Source: CAD feature listing. Evaluate the final solid. Frame: model axes, mm. Face numbers are marked on the shaded views. A direction names the side the tool comes from. Round coordinates to 2 decimals unless told otherwise and drop trailing zeros. Put each result on its own line as item: value.
```python
from build123d import *

# Parameters (mm, degrees)
SKETCH2_W               = 508
SKETCH2_H               = 127
BOSS_EXTRUDE1_DEPTH     = 63.5
SKETCH3_W               = 127
SKETCH3_H               = 127
BOSS_EXTRUDE2_DEPTH     = 444.5
SKETCH4_W               = 31.75
SKETCH4_H               = 31.75
CUT_EXTRUDE1_DEPTH      = 38.1
SKETCH5_R               = 12.7
CUT_EXTRUDE2_DEPTH      = 50.8
BOSS_EXTRUDE3_DEPTH     = 6.35
EXTRUDE_THIN1_START     = -6.35
EXTRUDE_THIN1_DEPTH     = 6.35
BOSS_EXTRUDE4_DEPTH     = 127
FILLET1_R               = 63.5
CUT_EXTRUDE3_DEPTH      = 583.156936495
CUT_EXTRUDE3_DEPTH_BACK = 583.156936495
SKETCH13_R              = 12.7


# Read off the part's stored shape, not the designer's step: Extrude-Thin1
with BuildPart() as part:
    # Sketch2 → Boss-Extrude1 (new body)
    with BuildSketch(Plane(origin=(0, 0, 0), x_dir=(0, 0, -1), z_dir=(1, 0, 0))):
        Rectangle(SKETCH2_W, SKETCH2_H)
    extrude(amount=BOSS_EXTRUDE1_DEPTH)

    # Sketch3 → Boss-Extrude2 (add)
    with BuildSketch(Plane(origin=(63.5, 0, 0), x_dir=(0, 0, -1), z_dir=(1, 0, 0))):
        Rectangle(SKETCH3_W, SKETCH3_H)
    extrude(amount=BOSS_EXTRUDE2_DEPTH)

    # Sketch4 → Cut-Extrude1 (cut)
    with BuildSketch(Plane.ZY):
        Rectangle(SKETCH4_W, SKETCH4_H)
    extrude(amount=-CUT_EXTRUDE1_DEPTH, mode=Mode.SUBTRACT)

    # Sketch5 → Cut-Extrude2 (cut)
    with BuildSketch(Plane.ZY.offset(-38.1)):
        Circle(SKETCH5_R)
    extrude(amount=-CUT_EXTRUDE2_DEPTH, mode=Mode.SUBTRACT)

    # Sketch10 → Boss-Extrude3 (add)
    with BuildSketch(Plane.XZ.offset(63.5)):
        Polygon((63.5, 254), (508, 63.5), (469.9, 63.5), (63.5, 237.671428571), align=None)
    boss_extrude3 = extrude(amount=-BOSS_EXTRUDE3_DEPTH)

    # Mirror1: Boss-Extrude3 across plane
    add(boss_extrude3.mirror(Plane.XY))

    # Extrude-Thin1 outline → Extrude-Thin1 (add)
    with BuildSketch(Plane(origin=(0, -57.15, 0), x_dir=(1, 0, 0), z_dir=(0, 1, 0)).offset(EXTRUDE_THIN1_START)):
        Polygon((82.952073355, -63.5), (76.2, -63.5), (278.373141881, -145.582939194), (281.657885075, -144.175192111), align=None)
        Polygon((266.7, -150.585714286), (63.5, -63.5), (63.5, -66.26343767), (263.475989385, -151.967433121), align=None)
        Polygon((255.026858119, -155.588489378), (63.5, -76.2), (63.5, -78.949557774), (251.765512342, -156.986208996), align=None)
    extrude_thin1 = extrude(amount=EXTRUDE_THIN1_DEPTH)

    # Mirror2: Extrude-Thin1 across plane
    add(extrude_thin1.mirror(Plane.XY))

    # Sketch12 → Boss-Extrude4 (add)
    with BuildSketch(Plane(origin=(0, 63.5, 0), x_dir=(1, 0, 0), z_dir=(0, 1, 0))):
        Polygon((508, 254), (508, 63.5), (571.5, 63.5), (571.5, 190.5), align=None)
        Polygon((571.5, 63.5), (508, 63.5), (508, -63.5), (508, -254), (571.5, -190.5), align=None)
    extrude(amount=-BOSS_EXTRUDE4_DEPTH)

    # Fillet1
    fillet1_edges = [part.edges().sort_by_distance(p)[0] for p in [
        (571.5, -63.5, 0),
        (571.5, 63.5, 0),
    ]]
    fillet(fillet1_edges, radius=FILLET1_R - 0.0001)  # a hair under: the kernel refuses the full size

    # Sketch13 → Cut-Extrude3 (cut, two sides: drawn at the far end of the back side and taken through both)
    with BuildSketch(Plane(origin=(106.321850008, -177.331865581, 0), x_dir=(0, 0, -1), z_dir=(-0.5142209424211187, 0.857657753638091, 0)).offset(-CUT_EXTRUDE3_DEPTH_BACK)):
        with Locations(Location((0, -341.343168692, 0), (0, 0, 90))):
            Circle(SKETCH13_R)
    extrude(amount=CUT_EXTRUDE3_DEPTH + CUT_EXTRUDE3_DEPTH_BACK, mode=Mode.SUBTRACT)


solid = part.part
```
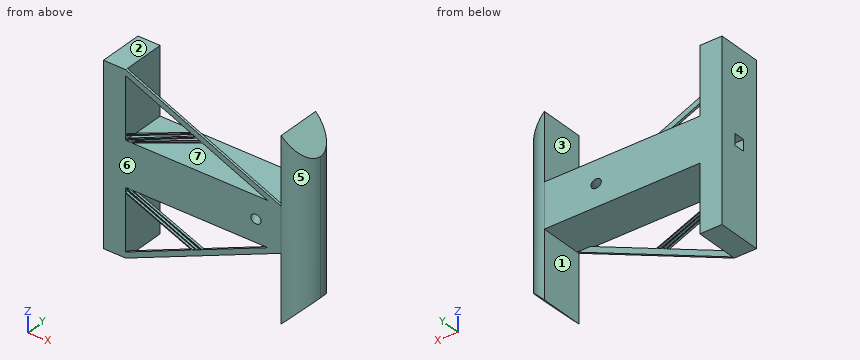
Q1. Cut plane B-B on x = 204. Give the number of separate pieces and of enclosed holes in the cut face, and give its area (3 significant figures).
Ans:
separate pieces: 9
enclosed holes: 0
area: 16,400 mm^2
Q2. Material intervals for line 1 (Z direction, x = 35, y = -11) (3 decimals); line 2 (Y direction, x = 62, z = 0); line 3 (X direction, y = 43, z = 85), sorted ascending. Write a range as [from, to].
Ans:
line 1: z = [-254, -15.875], [15.875, 254]
line 2: y = [-63.5, -12.7], [12.7, 63.5]
line 3: x = [0, 63.5], [508, 554.73]
Q3. Reachability of the marked faces 1, 2 and 3 from +Z, -Z, +X, -X, +Y, -Y: full face, straight path, thin tool, end or side. Return the list, or none.
Ans:
face 1: -Z, +Y, -Y
face 2: +Z, +X, -X, +Y, -Y
face 3: +Z, +Y, -Y
Q4. Draft query along X for the marked faces 4, 5, 6 and 7. Return one class per face: +X half, -X half, draft (parallel to the pull), parting line (faces both ways), or undercut.
Ans:
face 4: -X half
face 5: +X half
face 6: draft
face 7: undercut
Q5. Pin query (flat end, axial travel): pin 1 (3 mm diameter, centred on x = 233, y = 21, fed in from +Z); pin 2 (4 mm diameter, centred on x = 73.5, y = 29.5, fed in from -Z); pin 3 (12 mm diameter, centred on y = -27.5, z = -140, fed in from +X). Return the tip coordinate at first contact, or that it passes through.
Ans:
pin 1: stops at z = 63.5
pin 2: stops at z = -63.5
pin 3: stops at x = 567.75
